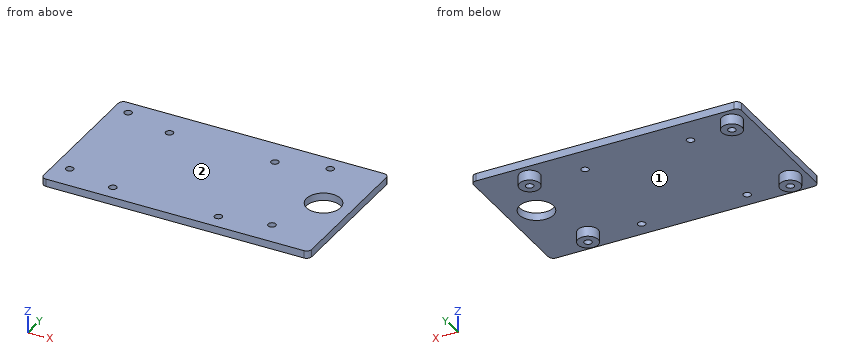
from build123d import *

# Parameters (mm, degrees)
SKETCH_R      = 1.5
SKETCH_R_2    = 6.75
PAD_DEPTH     = 3
SKETCH001_R   = 4
SKETCH001_R_2 = 1.5
PAD001_DEPTH  = 4
FILLET_R      = 2


with BuildPart() as part:
    # Sketch → Pad (new body)
    with BuildSketch(Plane.XY):
        Polygon((46, 27), (-46, 27), (-46, -28), (-46, -32), (60, -32), (60, -28), (60, 27), align=None)
        with Locations((20.85, 15.85)):
            Circle(SKETCH_R, mode=Mode.SUBTRACT)
        with Locations((-20.85, -25.85)):
            Circle(SKETCH_R, mode=Mode.SUBTRACT)
        with Locations((20.85, -25.85)):
            Circle(SKETCH_R, mode=Mode.SUBTRACT)
        with Locations((-20.85, 15.85)):
            Circle(SKETCH_R, mode=Mode.SUBTRACT)
        with Locations((48.85, -0.5)):
            Circle(SKETCH_R_2, mode=Mode.SUBTRACT)
        with Locations((-40, 21)):
            Circle(SKETCH_R, mode=Mode.SUBTRACT)
        with Locations((40, 21)):
            Circle(SKETCH_R, mode=Mode.SUBTRACT)
        with Locations((-40, -22)):
            Circle(SKETCH_R, mode=Mode.SUBTRACT)
        with Locations((40, -22)):
            Circle(SKETCH_R, mode=Mode.SUBTRACT)
    extrude(amount=PAD_DEPTH)

    # Sketch001 (on Face2 of Pad) → Pad001 (join)
    with BuildSketch(Plane(origin=(0, 0, 0), x_dir=(1, 0, 0), z_dir=(0, 0, -1))):
        with Locations((-40, 22)):
            Circle(SKETCH001_R)
        with Locations((-40, 22)):
            Circle(SKETCH001_R_2, mode=Mode.SUBTRACT)
        with Locations((40, 22)):
            Circle(SKETCH001_R)
        with Locations((40, 22)):
            Circle(SKETCH001_R_2, mode=Mode.SUBTRACT)
        with Locations((-40, -21)):
            Circle(SKETCH001_R)
        with Locations((-40, -21)):
            Circle(SKETCH001_R_2, mode=Mode.SUBTRACT)
        with Locations((40, -21)):
            Circle(SKETCH001_R)
        with Locations((40, -21)):
            Circle(SKETCH001_R_2, mode=Mode.SUBTRACT)
    extrude(amount=PAD001_DEPTH)

    # Fillet
    fillet_edges = [part.edges().sort_by_distance(p)[0] for p in [
        (-46, 27, 1.5),
        (-46, -32, 1.5),
        (60, -32, 1.5),
        (60, 27, 1.5),
    ]]
    fillet(fillet_edges, radius=FILLET_R)


solid = part.part
Here's how the part is built. I have some questions about the finished solid (model axes, mm). Face numbers are marked on the shaded views. Give positions to 0.01 mm unless a question says otherwise; leave off trailing zeros. Order: outer loops, then holes, each group sorted by start corner. A loop starts at its lowest first (then second) coordinate and runs counter-clockwise, first axis right, second up. Notation, with made-up numbers: (41.25, 70.5) -> (94.25, 70.5) arc R13 cw to (94.25, 87.5) -> close; hole circle Ø6 at (29, 2.25). An arc over 180 degrees is marked (long way). One line per item, written item: value. Start each with the question number.
1. Imagine slicing it at D-D, the plane z = 2. Count the separate pieces of the cut face and the enclosed holes in it, plus the area to 3 significant figures.
2. Imagine slicing it at C-C, the plane y = -0.5. List the corners of the cut face in (x, z) for me.
3. I need wall thicknesses on probe 1 along X at (y, z) = (-22, -0.75); probe 2 along Y at (x, z) = (20.85, 0.85); probe 3 along Y at (x, z) = (40, -1.75). Which ranges of each line are inside material? Lowest first, please. Write a range as from..to.
4. Will these pins go through, and if not, where does the flat tip stop? pin 1 Ø2.5 at (x, y) = (-20.85, -25.85) entering from -Z; pin 2 Ø10 at (x, y) = (17.5, 13.5) entering from -Z.
5. Imagine slicing it at A-A, the plane x = -20.85. List the corners of the cut face in (y, z) for me, plus the area to 3 significant figures.
6. We'd pull the mould along X, two halves only. Please class the marked faces 1 and 2: released by +X, released by -X, zero draft, split by the parting line, or undercut.
7. Imagine slicing it at B-B, the plane z = -3. List the corners of the cut face in (x, y) for me, plus the area to 3 significant figures.
Values follow:
1. separate pieces: 1
1. enclosed holes: 9
1. area: 6,050 mm2
2. outline: (-46, 0) -> (42.1, 0) -> (42.1, 3) -> (-46, 3) -> close; (55.6, 0) -> (60, 0) -> (60, 3) -> (55.6, 3) -> close
3. probe 1: x = -44..-41.5, -38.5..-36, 36..38.5, 41.5..44
3. probe 2: y = -32..-27.35, -24.35..14.35, 17.35..27
3. probe 3: y = -26..-23.5, -20.5..-18, 17..19.5, 22.5..25
4. pin 1: passes through
4. pin 2: stops at z = 0
5. outline: (-32, 0) -> (-27.35, 0) -> (-27.35, 3) -> (-32, 3) -> close; (-24.35, 0) -> (14.35, 0) -> (14.35, 3) -> (-24.35, 3) -> close; (17.35, 0) -> (27, 0) -> (27, 3) -> (17.35, 3) -> close
5. area: 159 mm2
6. face 1: undercut
6. face 2: zero draft
7. outline: circle Ø8 at (-40, -22); circle Ø8 at (-40, 21); circle Ø8 at (40, -22); circle Ø8 at (40, 21); hole circle Ø3 at (-40, -22); hole circle Ø3 at (-40, 21); hole circle Ø3 at (40, -22); hole circle Ø3 at (40, 21)
7. area: 173 mm2
